The model under review builds one solid part; all positions refer to its coordinate system, in mm. Face numbers are marked on the shaded views. Round coordinates to 2 decimals unless told otherwise and drop trailing zeros. Loops run counter-clockwise (first coordinate to the right, second up) from the corner with the lowest first, then second, coordinate; pieces in that order, holes last. Notation, with made-up numbers: M 21.5,76.25 L 68.5,76.25 A29 ccw 68.5,102.25 Z; hole C -9,86.5 d7. An arc over 180 degrees is marked long. Answer as a JSON object with one key per item and string values. Group by question number.
Item 1: The part is to be moulded in two halves that separate along X. For the marked faces 1 and 2, say which applies: +X half, -X half, draft (parallel to the pull), parting line (faces both ways), or undercut.
Item 2: Consider section C-C (x = 0). Give the boundary of the cut face in (y, z), and give its area (3 significant figures).
Item 3: Insertion check: P1, Ø1.8, axis at y = 14, z = 6.5, coming from the +X side; P2, Ø1.5, axis at y = -10.5, z = 5, coming from the -X side; P3, Ø4, axis at x = -3, z = 7.5, coming from the +Y side. Each pin has a flat end and moves straight along its axis. Give the tip position at first contact, or say it passes through.
Item 4: To check wall thickness, follow line 1 (X direction, y = 0, z = 8.85); line 2 (X direction, y = 0, z = 3.55); line 3 (Y direction, x = 0, z = 7.2). State the ranges of each line that lie inside material, in increasing order.
Item 5: Consider section A-A (x = 4.5). Give the boundary of the cut face in (y, z).
Item 6: Consider section B-B (y = -1). Give the boundary of the cut face in (x, z).
Item 7: Consider section D-D (z = 3.5). Give the boundary of the cut face in (x, y).
Autodesk Inventor part; units mm, degrees
ref_plane "YZ Plane" through (0, 0, 0) normal (1, 0, 0) x (0, 1, 0)
ref_plane "XZ Plane" through (0, 0, 0) normal (0, 1, 0) x (-1, 0, 0)
ref_plane "XY Plane" through (0, 0, 0) normal (0, 0, 1) x (1, 0, 0)
sketch "Sketch1" plane through (0, 0, 0) normal (0, 0, 1) x (1, 0, 0)
  circle A0 centre (0, 0) radius 12.45
  circle A1 centre (0, 0) radius 11
  circle A2 centre (0, 0) radius 15.6
  circle A3 centre (0, 0) radius 12
  dimension "d0" = 24.9
  dimension "d1" = 22
  dimension "d2" = 31.2
  dimension "d3" = 24
extrude "Extrusion1" add sketch "Sketch1" along normal blind 1 contours A3
extrude "Extrusion2" add sketch "Sketch1" along normal blind 4 contours A0
sketch "Sketch2" plane through (0, 0, 4) normal (0, 0, 1) x (1, 0, 0)
  circle A0 centre (0, 0) radius 15.6
  circle A1 centre (0, 0) radius 12
extrude "Extrusion3" add sketch "Sketch2" along normal blind 1
sketch "Sketch4" plane through (0, 0, 5) normal (0, 0, 1) x (1, 0, 0)
  circle A0 centre (0, 0) radius 16
  circle A1 centre (0, 0) radius 17
  circle A2 centre (0, 0) radius 12
  dimension "d14" = 32
  dimension "d15" = 34
extrude "Extrusion5" add sketch "Sketch4" along normal blind 0.5 contours A0
extrude "Extrusion6" add sketch "Sketch4" along normal blind 4 contours A1
sketch "Sketch5" plane through (0, 0, 9) normal (0, 0, 1) x (1, 0, 0)
  circle A0 centre (0, 0) radius 16
  circle A1 centre (0, 0) radius 15.5
  dimension "d20" = 31
extrude "Extrusion7" add sketch "Sketch5" against normal blind 0.25
sketch "Sketch8" plane through (0, 0, 9) normal (0, 0, 1) x (1, 0, 0)
  line L0 (0.5, 10) -> (-0.5, 10)
  line L1 (-0.5, 10) -> (-0.5, 20)
  line L2 (-0.5, 20) -> (0.5, 20)
  line L3 (0.5, 20) -> (0.5, 10)
  circle A0 centre (0, 0) radius 15
  line L4 (0.5, 10) -> (-0.5, 20) construction
  line L5 (-0.5, 10) -> (0.5, 20) construction
  point P0 (0, 15)
  dimension "d30" = 1
  dimension "d31" = 10
extrude "Extrusion10" cut sketch "Sketch8" against normal blind 10 contours L0 L1 A0 L3 | A0 L1 L2 L3 picked at (-0.0556, 11.6664)
properties part number "32mmFilterto25mmBoreAdapter"
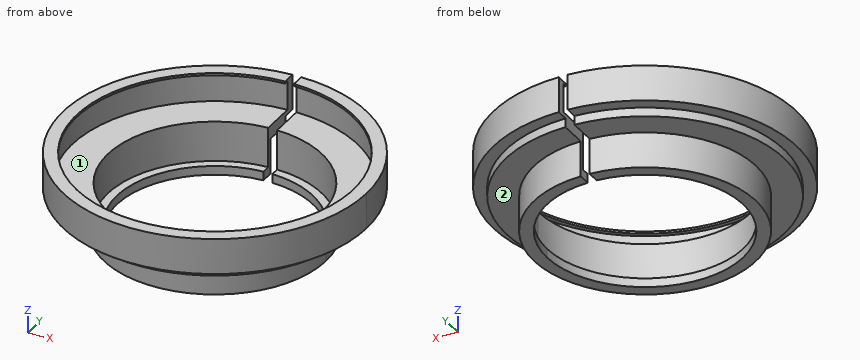
Geometry results:
{
 "1": {"face 1": "undercut", "face 2": "draft"},
 "2": {"outline": "M -17,5 L -15.6,5 L -15.6,4 L -12.45,4 L -12.45,0 L -11,0 L -11,1 L -12,1 L -12,5.5 L -16,5.5 L -16,8.75 L -15.5,8.75 L -15.5,9 L -17,9 Z", "area": "12.5 mm^2"},
 "3": {"P1": "stops at x = 10.83", "P2": "stops at x = -13.93", "P3": "stops at y = 16.97"},
 "4": {"line 1": "x = -17 to -15.5, 15.5 to 17", "line 2": "x = -12.45 to -12, 12 to 12.45", "line 3": "y = -17 to -16"},
 "5": {"outline": "M -16.39,5 L -14.94,5 L -14.94,4 L -11.61,4 L -11.61,0 L -10.04,0 L -10.04,1 L -11.12,1 L -11.12,5.5 L -15.35,5.5 L -15.35,8.75 L -14.83,8.75 L -14.83,9 L -16.39,9 Z; M 10.04,0 L 11.61,0 L 11.61,4 L 14.94,4 L 14.94,5 L 16.39,5 L 16.39,9 L 14.83,9 L 14.83,8.75 L 15.35,8.75 L 15.35,5.5 L 11.12,5.5 L 11.12,1 L 10.04,1 Z"},
 "6": {"outline": "M -16.97,5 L -15.57,5 L -15.57,4 L -12.41,4 L -12.41,0 L -10.95,0 L -10.95,1 L -11.96,1 L -11.96,5.5 L -15.97,5.5 L -15.97,8.75 L -15.47,8.75 L -15.47,9 L -16.97,9 Z; M 10.95,0 L 12.41,0 L 12.41,4 L 15.57,4 L 15.57,5 L 16.97,5 L 16.97,9 L 15.47,9 L 15.47,8.75 L 15.97,8.75 L 15.97,5.5 L 11.96,5.5 L 11.96,1 L 10.95,1 Z"},
 "7": {"outline": "M -0.5,11.99 L -0.5,12.44 A12.45 ccw long 0.5,12.44 L 0.5,11.99 A12 cw long Z"}
}
